The listing builds one solid part. Answer for the finished solid, in the listing's coordinates (mm). Face numbers are marked on the shaded views. A direction names the side the tool comes from. Give positions to 0.01 mm unless a question says otherwise; leave off trailing zeros. Write each loop counter-clockwise with the first axis right and the second up, starting at its lowest first coordinate (ties: lowest second). Pieces come first, ordered by that corner, then holes. Notation, with made-up numbers: (1, 61) - (30, 61) arc R28 ccw to (30, 87) - close; hole circle Ø7 at (40.5, 11.25). An arc over 180 degrees is marked (long way). One line per question, with ' | ' between items. Start each with the question number.
1. A cutting plane is placed at A-A (z = 0). Determine the outline of the cut face in (x, y).
2. Given P1, Ø23, axis at x = 23.5, y = 22.5, coming from the -Z side; P2, Ø11, axis at x = -64.5, z = -8, coming from the +Y side; P3, Ø20, axis at x = 0, y = 89, coming from the -Z side; P4, Ø10, axis at x = 23.5, z = 35, coming from the -Y side, each flat-ended and moving along its own axis, determine where each tip first touches the part or whether it passes through.
3. The mould has two halves that part along X. Classify the marked faces 4, 5, 6 and 7: +X half, -X half, draft (parallel to the pull), parting line (faces both ways), or undercut.
4. A cutting plane is placed at C-C (x = 15.5). Determine the outline of the cut face in (y, z), then the cut area to 3 significant figures.
5. A cutting plane is placed at D-D (y = 25.5). Determine the outline of the cut face in (x, z), then the cut area to 3 significant figures.
6. A cutting plane is placed at B-B (y = 11.5). Determine the outline of the cut face in (x, z).
7. For the marked faces 1, 2 and 3, determine the directions among +Z, -Z, +X, -X, +Y, -Y from which every point of the face is accessible in a straight line to the end or side of a thin tool.
8. Find the intervals of material crossed by L1, parallel to X at y = 4.75, z = 0; L2, parallel to X at y = 31, z = 0; L3, parallel to Y at x = -12, z = 100, in increasing order. Write a range as from..to.
```python
from build123d import *

# Parameters (mm, degrees)
CROQUIS2_R              = 18
CROQUIS2_R_2            = 9
SALIENTE_EXTRUIR1_DEPTH = 16
CROQUIS3_R              = 18
CROQUIS3_R_2            = 9
SALIENTE_EXTRUIR2_DEPTH = 19
CROQUIS4_R              = 35
CROQUIS4_R_2            = 18
SALIENTE_EXTRUIR3_DEPTH = 119
CROQUIS5_R              = 14
SALIENTE_EXTRUIR4_DEPTH = 37.5
SALIENTE_EXTRUIR5_DEPTH = 12
SALIENTE_EXTRUIR6_REACH = 195
CROQUIS7_R              = 24
CROQUIS7_R_2            = 12.5
CORTAR_EXTRUIR1_REACH   = 195
CROQUIS8_R              = 12.5


with BuildPart() as part:
    # Croquis2 → Saliente-Extruir1 (new body)
    with BuildSketch(Plane(origin=(0, 0, 0), x_dir=(1, 0, 0), z_dir=(0, 1, 0))):
        with BuildLine():
            Line((-65, 24), (-38.065732621, 24))
            ThreePointArc((-38.065732621, 24), (0, 45), (38.065732621, 24))
            Line((38.065732621, 24), (65, 24))
            ThreePointArc((65, 24), (87.272092101, 8.941695223), (81.595854962, -17.337173878))
            Line((81.595854962, -17.337173878), (37.5, -72))
            Line((37.5, -72), (-37.5, -72))
            Line((-37.5, -72), (-81.595854962, -17.337173878))
            ThreePointArc((-81.595854962, -17.337173878), (-87.272092101, 8.941695223), (-65, 24))
        make_face()
        Circle(CROQUIS2_R, mode=Mode.SUBTRACT)
        with Locations((65, 0)):
            Circle(CROQUIS2_R_2, mode=Mode.SUBTRACT)
        with Locations((-65, 0)):
            Circle(CROQUIS2_R_2, mode=Mode.SUBTRACT)
    extrude(amount=SALIENTE_EXTRUIR1_DEPTH)

    # Croquis3 → Saliente-Extruir2 (add)
    with BuildSketch(Plane(origin=(0, 0, 0), x_dir=(1, 0, 0), z_dir=(0, 1, 0))):
        with Locations((65, 0)):
            Circle(CROQUIS3_R)
        with Locations((65, 0)):
            Circle(CROQUIS3_R_2, mode=Mode.SUBTRACT)
        with Locations((-65, 0)):
            Circle(CROQUIS3_R)
        with Locations((-65, 0)):
            Circle(CROQUIS3_R_2, mode=Mode.SUBTRACT)
    extrude(amount=SALIENTE_EXTRUIR2_DEPTH)

    # Croquis4 → Saliente-Extruir3 (add)
    with BuildSketch(Plane(origin=(0, 0, 0), x_dir=(1, 0, 0), z_dir=(0, 1, 0))):
        Circle(CROQUIS4_R)
        Circle(CROQUIS4_R_2, mode=Mode.SUBTRACT)
    extrude(amount=SALIENTE_EXTRUIR3_DEPTH)

    # Croquis5 → Saliente-Extruir4 (add, symmetric)
    with BuildSketch(Plane(origin=(0, 0, 0), x_dir=(0, 0, -1), z_dir=(1, 0, 0))):
        with BuildLine():
            Line((-72, 0), (-72, 37))
            ThreePointArc((-72, 37), (-100, 65), (-128, 37))
            Line((-128, 37), (-128, 0))
            Line((-128, 0), (-72, 0))
        make_face()
        with Locations((-100, 37)):
            Circle(CROQUIS5_R, mode=Mode.SUBTRACT)
    extrude(amount=SALIENTE_EXTRUIR4_DEPTH, both=True)

    # Croquis6 → Saliente-Extruir5 (add)
    with BuildSketch(Plane(origin=(0, 0, 0), x_dir=(0, 0, -1), z_dir=(1, 0, 0))):
        with BuildLine():
            Line((-72, 16), (-18, 16))
            Line((-18, 16), (-18, 119))
            Line((-18, 119), (-35, 119))
            Line((-35, 119), (-116.487939559, 59.630683797))
            ThreePointArc((-116.487939559, 59.630683797), (-87.304770732, 61.95658538), (-72, 37))
            Line((-72, 37), (-72, 16))
        make_face()
    extrude(amount=SALIENTE_EXTRUIR5_DEPTH)

    # Croquis7 → Saliente-Extruir6 (add, up to next)
    with BuildSketch(Plane.XY.offset(-65), mode=Mode.PRIVATE) as saliente_extruir6_sk1:
        with Locations((0, 89)):
            Circle(CROQUIS7_R)
        with Locations((0, 89)):
            Circle(CROQUIS7_R_2, mode=Mode.SUBTRACT)
    saliente_extruir6_tool1 = extrude(saliente_extruir6_sk1.sketch, amount=SALIENTE_EXTRUIR6_REACH, mode=Mode.PRIVATE) - part.part
    add(saliente_extruir6_tool1.solids().sort_by_distance((-23.321177, 89, -65))[0])

    # Croquis8 → Cortar-Extruir1 (cut, up to next)
    with BuildSketch(Plane.XY.offset(-65), mode=Mode.PRIVATE) as cortar_extruir1_sk1:
        with Locations((0, 89)):
            Circle(CROQUIS8_R)
    cortar_extruir1_tool1 = extrude(cortar_extruir1_sk1.sketch, amount=CORTAR_EXTRUIR1_REACH, mode=Mode.PRIVATE) & part.part
    add(cortar_extruir1_tool1.solids().sort_by_distance((0, 89, -65))[0], mode=Mode.SUBTRACT)


solid = part.part
```
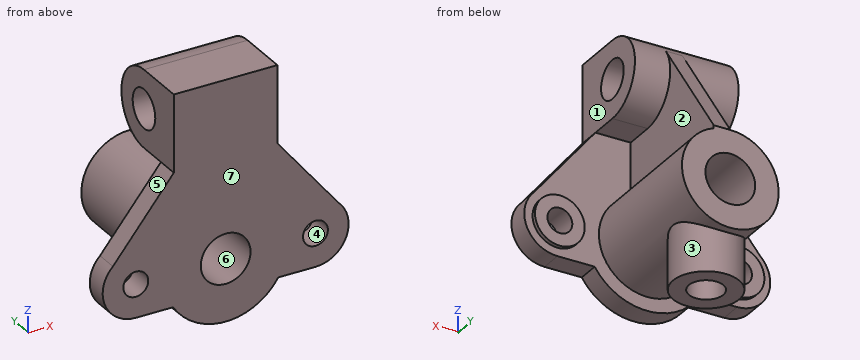
Determined:
1) outline: (-89, 0) - (-74, 0) - (-74, 19) - (-83, 19) - (-83, 16) - (-89, 16) - close; (-56, 0) - (-18, 0) - (-18, 119) - (-35, 119) - (-35, 16) - (-47, 16) - (-47, 19) - (-56, 19) - close; (18, 0) - (56, 0) - (56, 19) - (47, 19) - (47, 16) - (35, 16) - (35, 119) - (18, 119) - close; (74, 0) - (89, 0) - (89, 16) - (83, 16) - (83, 19) - (74, 19) - close
2) P1: z = -42.76 | P2: y = 19 | P3: z = 14.97 | P4: y = 0
3) face 4: undercut | face 5: -X half | face 6: undercut | face 7: draft
4) outline: (0, -42.25) - (16, -42.25) - (16, -31.38) - (70.68, -31.38) - (70.68, -65) - (107.32, -65) - (107.32, -31.38) - (119, -31.38) - (119, -9.15) - (0, -9.15) - close; (0, 9.15) - (119, 9.15) - (119, 31.38) - (16, 31.38) - (16, 72) - (37, 72) arc R28 ccw to (37, 128) - (0, 128) - close; hole circle Ø28 at (37, 100) | area: 10,000 mm2
5) outline: (-37.5, 72) - (0, 72) - (0, 35) arc R35 ccw (long way) to (12, 32.88) - (12, 72) - (37.5, 72) - (37.5, 92.02) - (-37.5, 92.02) - close; (-37.5, 107.98) - (37.5, 107.98) - (37.5, 128) - (-37.5, 128) - close; hole circle Ø36 at (0, 0) | area: 6,290 mm2
6) outline: (-81.6, 17.34) arc R24 ccw to (-65, -24) - (-38.07, -24) arc R45 ccw to (38.07, -24) - (65, -24) arc R24 ccw to (81.6, 17.34) - (37.5, 72) - (37.5, 128) - (-37.5, 128) - (-37.5, 72) - close; hole circle Ø18 at (-65, 0); hole circle Ø36 at (0, 0); hole circle Ø18 at (65, 0)
7) face 1: +Z, +X, +Y, -Y | face 2: +X, +Y | face 3: -Z
8) L1: -89..-74, -56..-18, 18..56, 74..89 | L2: -35..-18, 18..35 | L3: 0..23, 51..65
